Read the model definition and answer for the solid it produces. Units are mm, in the model's axes. A direction names the side the tool comes from. Give positions to 0.01 mm unless a question says otherwise; leave off trailing zeros. Write each loop counter-clockwise with the first axis right and the second up, starting at its lowest first coordinate (ties: lowest second). Pieces come first, ordered by that corner, then holes. Notation, with made-up numbers: M -31,51 L -4,51 A14 cw -4,68 Z; hole C 49.5,-11 d9. An arc over 180 degrees is marked long. Use a Markdown table: item, result. Add a question column.
Item 1: A cutting plane is placed at D-D on x = 3. Determine the outline of the cut face in (y, z), then the cut area to 3 significant figures.
Item 2: A cutting plane is placed at C-C on x = -60. Determine the outline of the cut face in (y, z), then the cut area to 3 significant figures.
Item 3: A cutting plane is placed at B-B on z = -60. Determine the outline of the cut face in (x, y).
Item 4: Given P1, Ø8, axis at x = 75, y = -35.5, coming from the +Z side; P2, Ø1.5, axis at x = 62, y = -66.5, coming from the +Z side, each flat-ended and moving along its own axis, determine where each tip first touches the part or whether it passes through.
Item 5: Consider probe 1 along X at (y, z) = (-112, -51); probe 2 along Y at (x, z) = (91.5, 37); probe 3 along X at (y, z) = (-93, 62). Determine where each line is inside the solid, lowest interval first. Write a range as [from, to].
Item 6: For faces 1 (the cylindrical face through (99, -2, -1)), 2 (the flat face through (-1, -20, -1)), determine the directions among +Z, -Z, +X, -X, +Y, -Y from which every point of the face is accessible in a straight line to the end or side of a thin tool.
Item 7: The mould has two halves that part along X. Classify faces 3 (the cylindrical face through (-66, -94, -68)), 4 (the flat face through (-60, -170, -60)), 5 (the cylindrical face through (-99, -2, -1)): pulls with the +X half, pulls with the -X half, needs draft (parallel to the pull), parting line crosses it, or undercut.
Item 8: A cutting plane is placed at A-A on y = -67. Determine the outline of the cut face in (x, z).
from build123d import *

# Parameters (mm, degrees)
SKETCH_1_W      = 200
SKETCH_1_H      = 200
EXTRUDE_1_DEPTH = 20
FILLET_1_R      = 5
SKETCH_4_R      = 10
EXTRUDE_4_DEPTH = 150


with BuildPart() as part:
    # 草图1 → 凸台-拉伸1 (new body)
    with BuildSketch(Plane(origin=(0, 0, 0), x_dir=(1, 0, 0), z_dir=(0, 1, 0))):
        Rectangle(SKETCH_1_W, SKETCH_1_H)
    extrude(amount=-EXTRUDE_1_DEPTH)

    # 圆角1
    fillet_1_edges = [part.edges().sort_by_distance(p)[0] for p in [
        (0, 0, -100),
        (100, 0, 0),
        (0, 0, 100),
        (-100, 0, 0),
    ]]
    fillet(fillet_1_edges, radius=FILLET_1_R)

    # 草图4 → 凸台-拉伸4 (add)
    with BuildSketch(Plane(origin=(0, -20, 0), x_dir=(1, 0, 0), z_dir=(0, 1, 0))):
        with Locations(Location((-60, 60, 0), (0, 0, 270))):
            Circle(SKETCH_4_R)
        with Locations(Location((60, 60, 0), (0, 0, 270))):
            Circle(SKETCH_4_R)
        with Locations(Location((-60, -60, 0), (0, 0, 270))):
            Circle(SKETCH_4_R)
        with Locations(Location((60, -60, 0), (0, 0, 270))):
            Circle(SKETCH_4_R)
    extrude(amount=-EXTRUDE_4_DEPTH)


solid = part.part
Filled in:
| question | item | result |
|---|---|---|
| 1 | outline | M -20,-100 L -5,-100 A5 ccw 0,-95 L 0,95 A5 ccw -5,100 L -20,100 Z |
| 1 | area | 3,990 mm² |
| 2 | outline | M -170,-70 L -20,-70 L -20,-100 L -5,-100 A5 ccw 0,-95 L 0,95 A5 ccw -5,100 L -20,100 L -20,70 L -170,70 L -170,50 L -20,50 L -20,-50 L -170,-50 Z |
| 2 | area | 9,990 mm² |
| 3 | outline | M -100,-20 L -70,-20 L -70,-170 L -50,-170 L -50,-20 L 50,-20 L 50,-170 L 70,-170 L 70,-20 L 100,-20 L 100,-5 A5 ccw 95,0 L -95,0 A5 ccw -100,-5 Z |
| 4 | P1 | through |
| 4 | P2 | z = 69.92 |
| 5 | probe 1 | [-64.36, -55.64], [55.64, 64.36] |
| 5 | probe 2 | [-20, 0] |
| 5 | probe 3 | [-69.8, -50.2], [50.2, 69.8] |
| 6 | face 1 | +Z, -Z, +X, +Y |
| 6 | face 2 | -Y |
| 7 | face 3 | undercut |
| 7 | face 4 | needs draft |
| 7 | face 5 | pulls with the -X half |
| 8 | outline | C -60,-60 d20; C -60,60 d20; C 60,-60 d20; C 60,60 d20 |
